Autodesk Fusion 360 part; units mm, degrees
sketch "スケッチ1" plane through (0, 0, 0) normal (0, 1, 0) x (1, 0, 0)
  line L0 (-25, -10) -> (25, -10)
  arc A0 (25, -10) -> (25, 10) centre (25, 0) ccw
  line L1 (25, 10) -> (-25, 10)
  arc A1 (-25, 10) -> (-25, -10) centre (-25, 0) ccw
  line L2 (-25, 0) -> (25, 0) construction
  line L3 (-23, 10) -> (-23, -10) construction
  line L4 (-15, 10) -> (-15, -10) construction
  line L5 (15, 10) -> (15, -10) construction
  line L6 (23, 10) -> (23, -10) construction
  line L7 (-23, -1) -> (23, -1) construction
  line L8 (-15, -2) -> (15, -2) construction
  line L9 (0, 10) -> (0, -10) construction
  line L10 (-24.25, -0.25) -> (-24.25, -1.75)
  arc A2 (-24.25, -1.75) -> (-21.75, -1.75) centre (-23, -1.75) ccw
  line L11 (-21.75, -1.75) -> (-21.75, -0.25)
  arc A3 (-21.75, -0.25) -> (-24.25, -0.25) centre (-23, -0.25) ccw
  line L12 (-23, -0.25) -> (-23, -1.75) construction
  point P0 (-35, 0)
  point P1 (35, 0)
  point P2 (-23, -1)
  point P3 (-15, -2)
  point P4 (15, -2)
  point P5 (23, -1)
  point P6 (0, 2)
  point P7 (0, -4)
  point P8 (-23, -1)
  point P9 (-23, 1)
  point P10 (-23, -3)
  dimension "d1" = 20
  dimension "d2" = 70
  dimension "d13" = 6
  dimension "d14" = 12
  dimension "d15" = 9
  dimension "d16" = 8
  dimension "d17" = 15
  dimension "d18" = 15
  dimension "d19" = 23
  dimension "d20" = 23
  dimension "d40" = 4
  dimension "d41" = 2.5
extrude "押し出し1" add sketch "スケッチ1" along normal blind 3 contours L0 A0 L1 A1 | L10 A2 L11 A3
chamfer "面取り1" distance 1 angle 45 4 edges at (0, 3, -10) (-35, 3, 0) (0, 3, 10) (35, 3, 0)
sketch "スケッチ2" plane through (0, 3, 0) normal (0, 1, 0) x (-1, 0, 0)
  line L0 (-25, -9) -> (25, -9)
  arc A0 (25, -9) -> (25, 9) centre (25, 0) ccw
  line L1 (25, 9) -> (-25, 9)
  arc A1 (-25, 9) -> (-25, -9) centre (-25, 0) ccw
  arc A2 (25, -10) -> (25, 10) centre (25, 0) ccw
  line L2 (-25, -10) -> (25, -10)
  arc A3 (-25, 10) -> (-25, -10) centre (-25, 0) ccw
  line L3 (25, 10) -> (-25, 10)
  line L4 (35, 0) -> (-35, 0) construction
  point P0 (29.8, 0)
  point P1 (-29.8, 0)
  dimension "d6" = 5.2
  dimension "d7" = 5.2
hole "穴1" at (-29.8, 3, 0) at (29.8, 3, 0) direction (0, -1, 0) diameter 3.5 end through all countersink diameter 6.8 countersink angle 90
hole "穴2" at (0, 0, -2) direction (0, 1, 0) diameter 7.5 end through all
hole "穴3" at (0, 0, 4) direction (0, 1, 0) diameter 2 depth 1 tip angle 180
hole "穴4" at (-15, 0, 2) at (15, 0, 2) direction (0, 1, 0) diameter 5.5 end through all counterbore diameter 10 counterbore depth 1.5
hole "穴5" at (-23, 0, 1) direction (0, 1, 0) diameter 4 end through all counterbore diameter 9 counterbore depth 1.5
hole "穴6" at (23, 0, 1) direction (0, 1, 0) diameter 3.5 end through all
Model file for the job. Use its own axes, mm. A direction names the side the tool comes from. Give positions to 0.01 mm unless a question says otherwise; leave off trailing zeros. Loops run counter-clockwise (first coordinate to the right, second up) from the corner with the lowest first, then second, coordinate; pieces in that order, holes last. Notation, with made-up numbers: (-3, 62.25) -> (40, 62.25) arc R22 ccw to (40, 98.25) -> close; hole circle Ø8 at (-21.75, -1.5). An arc over 180 degrees is marked (long way). Use a Markdown table: item, result. Add a question column.
(1) Slice it at C-C on x = -11. List the corners of the cut face in (y, z).
(2) Wall check: line 1 along Z through (x, y) = (15, 0.5); line 2 along X through (y, z) = (0.45, 2.5); line 3 along Y through (x, z) = (-13.5, -1.75). Give the ranges that are in metal, low to high.
(3) Slice it at B-B on y = 2.5. List the corners of the cut face in (x, z).
(4) Mould opens along X. For faces 1 (the conical face through (34.2, 2.8, -0.2)), 2 (the flat face through (0, 3, 2)), 3 (the conical face through (-29.2, 1.5, 1.8)), 4 (the cylindrical face through (19.88, 0.76, 3.08)) say: +X half, -X half, draft (parallel to the pull), parting line (faces both ways), or undercut.
(5) Drop flat-ended pins along their axis: pin 1 Ø3 at (x, z) = (23, 1) entering from -Y; pin 2 Ø4.5 at (x, z) = (-29.8, 0) entering from +Y; pin 3 Ø1 at (y, z) = (0.5, 5) entering from +X; pin 4 Ø6.5 at (x, z) = (-23, 1) entering from -Y. Give the stop position or say it passes through.
(6) Slice it at D-D on x = -23. List the corners of the cut face in (y, z), and give its area (3 significant figures).
(7) Slice it at A-A on x = 15. List the corners of the cut face in (y, z).
(8) Tool access for faces 5 (the flat face through (0, 1, 10)), 6 (the flat face through (0, 1, 4)): list every direction of +Z, -Z, +X, -X, +Y, -Y with a clear straight run to the whole face (end or side of a thin tool).
Filled sheet:
| question | item | result |
|---|---|---|
| 1 | outline | (0, -10) -> (2, -10) -> (3, -9) -> (3, 9) -> (2, 10) -> (0, 10) -> (0, 5) -> (1.5, 5) -> (1.5, -1) -> (0, -1) -> close |
| 2 | line 1 | -10 to -3, 7 to 10 |
| 2 | line 2 | -34.68 to -27.24, -10.03 to 10.03, 19.97 to 22.1, 23.9 to 34.68 |
| 2 | line 3 | 1.5 to 3 |
| 3 | outline | (-25, -9.5) -> (25, -9.5) arc R9.5 ccw to (25, 9.5) -> (-25, 9.5) arc R9.5 ccw to start; hole circle Ø5.8 at (-29.8, 0); hole circle Ø4 at (-23, 1); hole circle Ø5.5 at (-15, 2); hole circle Ø7.5 at (0, -2); hole circle Ø5.5 at (15, 2); hole circle Ø3.5 at (23, 1); hole circle Ø5.8 at (29.8, 0) |
| 4 | face 1 | +X half |
| 4 | face 2 | draft |
| 4 | face 3 | undercut |
| 4 | face 4 | undercut |
| 5 | pin 1 | through |
| 5 | pin 2 | y = 1.85 |
| 5 | pin 3 | x = 33.93 |
| 5 | pin 4 | y = 1.5 |
| 6 | outline | (0, -10) -> (2, -10) -> (3, -9) -> (3, -1) -> (1.5, -1) -> (1.5, -3.5) -> (0, -3.5) -> close; (0, 5.5) -> (1.5, 5.5) -> (1.5, 3) -> (3, 3) -> (3, 9) -> (2, 10) -> (0, 10) -> close |
| 6 | area | 39.5 mm2 |
| 7 | outline | (0, -10) -> (2, -10) -> (3, -9) -> (3, -0.75) -> (1.5, -0.75) -> (1.5, -3) -> (0, -3) -> close; (0, 7) -> (1.5, 7) -> (1.5, 4.75) -> (3, 4.75) -> (3, 9) -> (2, 10) -> (0, 10) -> close |
| 8 | face 5 | +Z, +X, -X, +Y, -Y |
| 8 | face 6 | -Y |
